from build123d import *

# Parameters (mm, degrees)
SKETCH1_W           = 50
SKETCH1_H           = 11
BOSS_EXTRUDE1_DEPTH = 8
FILLET1_R           = 20
FILLET2_R           = 8
SKETCH2_R           = 3.25
CUT_EXTRUDE1_DEPTH  = 21


# Some blends are built 0.0001 mm under size
with BuildPart() as part:
    # Sketch1 → Boss-Extrude1 (new body)
    with BuildSketch(Plane(origin=(0, 0, 0), x_dir=(1, 0, 0), z_dir=(0, 1, 0))):
        Rectangle(SKETCH1_W, SKETCH1_H)
    extrude(amount=BOSS_EXTRUDE1_DEPTH)

    # Fillet1
    # the kernel refuses this fillet: 20 mm, written as the material it takes off along each edge
    with BuildSketch(Plane(origin=(-25, 0, -45.5), x_dir=(0, 1, 0), z_dir=(0, 0, 1))) as fillet1_piece_1:
        with BuildLine():
            CenterArc((20, -16), FILLET1_R, 126.869897646, 53.130102354)
            Line((0, -16), (-0.4, -16))
            Line((-0.4, -16), (-0.4, 0))
            Line((-0.4, 0), (0, 0.4))
            ThreePointArc((0, 0.4), (4, 0.4), (7.76, 0.32))
            Line((7.76, 0.32), (8, 0))
        make_face()
    extrude(amount=91, mode=Mode.SUBTRACT)

    # Fillet2
    fillet2_edges = [part.edges().sort_by_distance(p)[0] for p in [
        (25, 0, 0),
    ]]
    fillet(fillet2_edges, radius=FILLET2_R - 0.0001)  # a hair under: the kernel refuses the full size

    # Sketch2 → Cut-Extrude1 (cut)
    with BuildSketch(Plane.XY.offset(5.5)):
        with Locations((0, 4)):
            Circle(SKETCH2_R)
    extrude(amount=-CUT_EXTRUDE1_DEPTH, mode=Mode.SUBTRACT)


solid = part.part
Geometry: final body of the model. Coordinates: model frame, mm. Coordinates: 2 decimals unless noted, no trailing zeros. Loops run counter-clockwise (first coordinate to the right, second up) from the corner with the lowest first, then second, coordinate; pieces in that order, holes last. Notation, with made-up numbers: (24.5, 28) - (50.5, 28) arc R22 ccw to (50.5, 42) - close; hole circle Ø6 at (68, -5.75). An arc over 180 degrees is marked (long way). Put each result on its own line as item: value. Start each with the question number.
Q1. Cut plane D-D, the plane x = 20. Return loops of the section in (y, z).
Q2. Pull-direction query (Y, two-part tool) for faces 1 (the flat face through (0, 8, 0)), 2 (the cylindrical face through (-0.423, 7.222, 0.077)), 3 (the cylindrical face through (22.719, 2.406, -0.077)), 4 (the flat face through (5, 4, -5.5)); classes: released by +Y, released by -Y, zero draft, split by the parting line, or undercut.
Q3. Pin query (flat end, axial travel): pin 1 Ø1 at (y, z) = (4.5, -4) entering from +X; pin 2 Ø2 at (y, z) = (4.5, -2.5) entering from -X (3 decimals); pin 3 Ø4 at (y, z) = (6.5, 4) entering from -X. Return the tip coordinate at first contact, or that it passes through.
Q4. Cut plane B-B, the plane y = 5.5. Return loops of the section in (x, z).
Q5. Line query: line 1 (Y direction, x = 0, z = 0); line 2 (X direction, y = 3.5, z = -2.5); line 3 (X direction, y = 1.75, z = 4). Output: solid intervals per line, ascending.
Q6. Cut plane A-A, the plane x = 0. Return loops of the section in (y, z), and give its area (3 significant figures).
Filled sheet:
1. outline: (0.58, -5.5) - (8, -5.5) - (8, 5.5) - (0.58, 5.5) - close
2. face 1: released by +Y
2. face 2: undercut
2. face 3: released by -Y
2. face 4: zero draft
3. pin 1: x = 24.42
3. pin 2: x = -22.775
3. pin 3: x = -25
4. outline: (-22.77, -5.5) - (-2.88, -5.5) - (-2.88, 5.5) - (-22.77, 5.5) - close; (2.88, -5.5) - (24.6, -5.5) - (24.6, 5.5) - (2.88, 5.5) - close
5. line 1: 0 to 0.75, 7.25 to 8
5. line 2: -20.3 to -3.21, 3.21 to 23.61
5. line 3: -17.18 to -2.35, 2.35 to 21.99
6. outline: (0, -5.5) - (0.75, -5.5) - (0.75, 5.5) - (0, 5.5) - close; (7.25, -5.5) - (8, -5.5) - (8, 5.5) - (7.25, 5.5) - close
6. area: 16.5 mm²
